from build123d import *

# Parameters (mm, degrees)
F0_W     = 76.2
F0_H     = 76.2
F1_DEPTH = 25.4
F3_DEPTH = 12.7


with BuildPart() as f1:
    # F0 (on Front) → F1 (new body)
    with BuildSketch(Plane.XZ):
        with Locations((0.062458, -9.009712)):
            Rectangle(F0_W, F0_H)
    extrude(amount=F1_DEPTH)

    # F2 (on face) → F3 (cut)
    with BuildSketch(Plane.XZ.offset(25.4)):
        Polygon((-29.074673, -43.174796), (-29.074673, -47.109712), (-21.642048, -47.109712), (-21.642048, -38.584057), (-6.558197, -38.584057), (-6.558197, -44.923648), (33.884019, -44.923648), (33.884019, -11.258238), (26.888607, -10.602417), (26.888607, -41.425943), (0, -41.425943), (0, -38.584057), (8.525654, -38.584057), (8.525654, -31.807255), (18.144343, -31.807255), (18.144343, -27.216518), (3.279097, -27.216518), (3.279097, -35.414262), (-21.642048, -35.414262), (-21.642048, -23.718812), (3.934919, -23.718812), (3.934919, -18.690862), (21.204835, -18.690862), (21.204835, -13.881517), (3.934919, -13.881517), (3.934919, -7.760533), (21.64205, -7.760533), (21.64205, 2.295369), (35.851475, 2.295369), (35.851475, 8.197745), (33.665411, 8.197745), (33.665411, 24.811845), (27.544426, 24.811845), (27.544426, 8.197745), (14.865247, 8.197745), (14.865247, -2.951189), (3.934919, -2.951189), (3.934919, 5.355861), (-16.395492, 5.355861), (-16.395492, 13.225697), (25.35836, 13.225697), (25.35836, 29.090288), (18.144343, 29.090288), (18.144343, 18.909467), (-24.265327, 18.909467), (-24.265327, 14.31873), (-27.981639, 14.31873), (-27.981639, 21.532746), (14.865247, 21.532746), (14.865247, 27.216518), (-34.977049, 27.216518), (-34.977049, 8.197745), (-24.265327, 8.197745), (-24.265327, 0), (-1.967459, 0), (-1.967459, -1.639549), (-30.823525, -1.639549), (-30.823525, -6.6675), (-1.967459, -6.6675), (-1.967459, -17.597828), (-29.074673, -17.597828), (-29.074673, -38.584057), (-31.916559, -38.584057), (-31.916559, -14.100123), (-6.339591, -14.100123), (-5.683769, -9.509386), (-36.507297, -9.509386), (-36.507297, -43.174796), align=None)
        with BuildLine():
            Line((2e-06, 61.738352), (0, 55.198155))
            ThreePointArc((0, 55.198155), (1.854865, 58.468253), (2e-06, 61.738352))
        make_face()
    extrude(amount=-F3_DEPTH, mode=Mode.SUBTRACT)


solid = f1.part
Model file for the job. Use its own axes, mm. A direction names the side the tool comes from. Round coordinates to 2 decimals unless told otherwise and drop trailing zeros. Order: outer loops, then holes, each group sorted by start corner. A loop starts at its lowest first (then second) coordinate and runs counter-clockwise, first axis right, second up.
(1) Band-saw the part on C-C (z = 11.5). List the corners of the cut face in (x, y), then the cut area to 3 significant figures.
(2) Drill centre lines: line 1 (Z direction, x = 19, y = -15.75); line 2 (X direction, y = -23.5, z = 10); line 3 (X direction, y = -18.75, z = 14.5). Where is each one in solid material? Low to high.
(3) Band-saw the part on A-A (z = -34.5). List the corners of the cut face in (x, y).
(4) 3-axis set-ups, long thin cutter, end or side, ignore diameter. For faces 1 (the face through (-21.642, -19, -30)), 2 (the face through (3.935, -19, 1)): which of +Z, -Z, +X, -X, +Y, -Y reach the whole face in a straight line?
(5) Band-saw the part on D-D (x = -1). List the corners of the cut face in (y, z), then the cut area to 3 significant figures.
(6) Band-saw the part on B-B (x = -26.5). List the corners of the cut face in (y, z).
(7) Pull direction X, two halves, no side cores. Call faces 3 (the face through (14, -25.4, -8)), 4 (the face through (-6, -19, 5.356)), 5 (the face through (18.144, -19, -30)), 6 (the face through (38.162, -13, -10)): released by +X, released by -X, zero draft, split by the parting line, or undercut.
Verdict:
1. outline: (-38.04, -25.4) - (-34.98, -25.4) - (-34.98, -12.7) - (-16.4, -12.7) - (-16.4, -25.4) - (27.54, -25.4) - (27.54, -12.7) - (33.67, -12.7) - (33.67, -25.4) - (38.16, -25.4) - (38.16, 0) - (-38.04, 0) - close
1. area: 1,620 mm2
2. line 1: z = -47.11 to -44.92, -41.43 to -18.69, -13.88 to -7.76, 8.2 to 13.23
2. line 2: x = -38.04 to -34.98, -16.4 to 27.54, 33.67 to 38.16
2. line 3: x = -38.04 to -34.98, -27.98 to -24.27, 25.36 to 27.54, 33.67 to 38.16
3. outline: (-38.04, -25.4) - (-36.51, -25.4) - (-36.51, -12.7) - (-31.92, -12.7) - (-31.92, -25.4) - (-29.07, -25.4) - (-29.07, -12.7) - (-21.64, -12.7) - (-21.64, -25.4) - (3.28, -25.4) - (3.28, -12.7) - (8.53, -12.7) - (8.53, -25.4) - (26.89, -25.4) - (26.89, -12.7) - (33.88, -12.7) - (33.88, -25.4) - (38.16, -25.4) - (38.16, 0) - (-38.04, 0) - close
4. face 1: -Z, -Y
4. face 2: -Y
5. outline: (-25.4, -47.11) - (0, -47.11) - (0, 29.09) - (-25.4, 29.09) - (-25.4, 27.22) - (-12.7, 27.22) - (-12.7, 21.53) - (-25.4, 21.53) - (-25.4, 18.91) - (-12.7, 18.91) - (-12.7, 13.23) - (-25.4, 13.23) - (-25.4, 5.36) - (-12.7, 5.36) - (-12.7, -23.72) - (-25.4, -23.72) - (-25.4, -35.41) - (-12.7, -35.41) - (-12.7, -44.92) - (-25.4, -44.92) - close
5. area: 1,300 mm2
6. outline: (-25.4, -17.6) - (-12.7, -17.6) - (-12.7, -47.11) - (0, -47.11) - (0, 29.09) - (-25.4, 29.09) - (-25.4, 27.22) - (-12.7, 27.22) - (-12.7, 21.53) - (-25.4, 21.53) - (-25.4, 14.32) - (-12.7, 14.32) - (-12.7, 8.2) - (-25.4, 8.2) - (-25.4, -1.64) - (-12.7, -1.64) - (-12.7, -6.67) - (-25.4, -6.67) - (-25.4, -9.51) - (-12.7, -9.51) - (-12.7, -14.1) - (-25.4, -14.1) - close
7. face 3: zero draft
7. face 4: undercut
7. face 5: undercut
7. face 6: released by +X
